Can you work these out from the model? Positions are in its coordinate system, mm. A direction names the side the tool comes from. Round coordinates to 2 decimals unless told otherwise and drop trailing zeros. Write each loop counter-clockwise with the first axis right and the second up, starting at its lowest first coordinate (ties: lowest second). Pieces come first, ordered by that corner, then holes. Notation, with made-up numbers: M 74.5,21.25 L 112.5,21.25 A24 ccw 112.5,47.25 Z; hole C 87,42.25 d3. An arc over 180 degrees is marked long. Answer in a Markdown table with one row per item. Add a question column.
(1) If I drill on probe 1 along X at (y, z) = (-1.5, 0); probe 2 along Y at (x, z) = (4.75, 3); probe 3 along X at (y, z) = (-2.5, -2.75), over which ranges is the centre line in solid material (lowest first)?
(2) Suppose I cut it at B-B, the plane z = -0.25. Write out the boundary of the cut face in (x, y), then the cut area to 3 significant figures.
(3) Suppose I cut it at D-D, the plane y = 2.25. Write out the boundary of the cut face in (x, z), then the cut area to 3 significant figures.
(4) Suppose I cut it at A-A, the plane x = 0. Write out the boundary of the cut face in (y, z).
(5) I'm going to push flat-ended pins straight in: pin 1 (5 mm diameter, centred on x = 2.5, y = 3.5, fed in from -Z); pin 2 (6 mm diameter, centred on y = 3.5, z = -4, fed in from -X); pin 3 (8 mm diameter, centred on x = 1.5, z = 0.5, fed in from -Y); pin 4 (4 mm diameter, centred on y = 4.5, z = 1.5, fed in from +X). Where does each tip first touch, or does it pass through?
(6) If we mould it in two halves opening along Z, with no side actions, what happens to faces 1 (the face through (-2.4, 5.5, 2.4)), 2 (the face through (0.9, 0.08, 2.86)), 3 (the face through (0.33, -5.007, 7.493))? For each: released by +Z, released by -Z, zero draft, split by the parting line, or undercut.
(7) For faces 4 (the face through (4, -4.5, 4)), 5 (the face through (0.1, -5.5, -3.2)), which set-ups out of +Z, -Z, +X, -X, +Y, -Y let a thin tool reach every point of the face, with its end or its side?
(8) Suppose I cut it at C-C, the plane x = 4. Write out the boundary of the cut face in (y, z).
from build123d import *

# Parameters (mm, degrees)
SKETCH1_R           = 5.5
BOSS_EXTRUDE1_DEPTH = 5.5
SKETCH2_R           = 7.5
BOSS_EXTRUDE2_DEPTH = 1
SKETCH3_R           = 3
CUT_EXTRUDE1_DEPTH  = 16.28070679


with BuildPart() as part:
    # Sketch1 → Boss-Extrude1 (new, symmetric)
    with BuildSketch(Plane(origin=(0, 0, 0), x_dir=(1, 0, 0), z_dir=(0, 1, 0))):
        with Locations(Location((0, 0, 0), (0, 0, 270))):
            Circle(SKETCH1_R)
    extrude(amount=BOSS_EXTRUDE1_DEPTH, both=True)

    # Sketch2 → Boss-Extrude2 (add)
    with BuildSketch(Plane.XZ.offset(5.5)):
        with Locations(Location((0, 0, 0), (0, 0, 270))):
            Circle(SKETCH2_R)
    extrude(amount=-BOSS_EXTRUDE2_DEPTH)

    # Sketch3 → Cut-Extrude1 (cut, through all)
    with BuildSketch(Plane(origin=(0, 5.5, 0), x_dir=(1, 0, 0), z_dir=(0, 1, 0))):
        with Locations(Location((0, 0, 0), (0, 0, 270))):
            Circle(SKETCH3_R)
    extrude(amount=-CUT_EXTRUDE1_DEPTH, mode=Mode.SUBTRACT)


solid = part.part
Calculated:
| question | item | result |
|---|---|---|
| 1 | probe 1 | -5.5 to -3, 3 to 5.5 |
| 1 | probe 2 | -5.5 to -4.5 |
| 1 | probe 3 | -4.76 to -1.2, 1.2 to 4.76 |
| 2 | outline | M -7.5,-5.5 L -2.99,-5.5 L -2.99,5.5 L -5.49,5.5 L -5.49,-4.5 L -7.5,-4.5 Z; M 2.99,-5.5 L 7.5,-5.5 L 7.5,-4.5 L 5.49,-4.5 L 5.49,5.5 L 2.99,5.5 Z |
| 2 | area | 59.1 mm² |
| 3 | outline | C 0,0 d11; hole C 0,0 d6 |
| 3 | area | 66.8 mm² |
| 4 | outline | M -5.5,-7.5 L -4.5,-7.5 L -4.5,-5.5 L 5.5,-5.5 L 5.5,-3 L -5.5,-3 Z; M -5.5,3 L 5.5,3 L 5.5,5.5 L -4.5,5.5 L -4.5,7.5 L -5.5,7.5 Z |
| 5 | pin 1 | z = -5.5 |
| 5 | pin 2 | x = -5.41 |
| 5 | pin 3 | y = -5.5 |
| 5 | pin 4 | x = 5.5 |
| 6 | face 1 | zero draft |
| 6 | face 2 | undercut |
| 6 | face 3 | split by the parting line |
| 7 | face 4 | +Y |
| 7 | face 5 | +Z, -Z, +X, -X, -Y |
| 8 | outline | M -5.5,-6.34 L -4.5,-6.34 L -4.5,-3.77 L 5.5,-3.77 L 5.5,3.77 L -4.5,3.77 L -4.5,6.34 L -5.5,6.34 Z |
